Autodesk Inventor part; units mm, degrees
ref_plane "YZ Plane" through (0, 0, 0) normal (1, 0, 0) x (0, 1, 0)
ref_plane "XZ Plane" through (0, 0, 0) normal (0, 1, 0) x (-1, 0, 0)
ref_plane "XY Plane" through (0, 0, 0) normal (0, 0, 1) x (1, 0, 0)
sketch "Sketch1" plane through (0, 0, 0) normal (0, 0, 1) x (1, 0, 0)
  arc A0 (62.3383, -89.7392) -> (-62.3386, -89.7387) centre (0.0001, -5.2464) ccw
  arc A1 (61.8662, -89.0928) -> (-61.866, -89.0928) centre (0.0001, -5.2464) ccw
  line L0 (-62.3386, -89.7387) -> (-61.866, -89.0928)
  line L1 (62.3383, -89.7392) -> (61.8662, -89.0928)
  point P0 (0, 0)
  dimension "d0" = 208.4
extrude "Extrusion1" add sketch "Sketch1" along normal blind 30
ref_plane "Work Plane1" through (61.0727, -89.6701, 0) normal (0.6382, -0.7699, 0) x (0.7699, 0.6382, 0)
sketch "Sketch2" plane through (61.0727, -89.6701, 0) normal (0.6382, -0.7699, 0) x (0.7699, 0.6382, 0)
  circle A0 centre (6.5, 25.5) radius 1.4
  circle A1 centre (6.5, 4.5) radius 1.4
  point P0 (10.2035, 0)
extrude "Extrusion2" cut sketch "Sketch2" along normal blind 30
mirror "Mirror1" about plane through (0, 0, 0) normal (1, 0, 0) of "Extrusion2"
properties part number "3rdShroud"
Model file for the job. Use its own axes, mm. Give positions to 0.01 mm unless a question says otherwise; leave off trailing zeros. Loops run counter-clockwise (first coordinate to the right, second up) from the corner with the lowest first, then second, coordinate; pieces in that order, holes last.
Item 1: Slice it at D-D (x = 42.5). Write the cut outline in (y, z).
Check values:
outline: (89.89, 0) - (90.77, 0) - (90.77, 30) - (89.89, 30) - close
Item 2: Drop flat-ended pins along their axis: P1, Ø1, axis at x = -81.5, z = 23.5, coming from the -Y side; P2, Ø3, axis at y = 5.5, z = 19.5, coming from the -X side; P3, Ø8, axis at y = 4.5, z = 5.5, coming from the -X side. Give the stop position or say it passes through.
Check values:
P1: stops at y = -72.06
P2: stops at x = -104.59
P3: stops at x = -104.84
Item 3: Slice it at B-B (y = 35.5). Write the cut outline in (x, z).
Check values:
outline: (-96.77, 0) - (-95.9, 0) - (-95.9, 30) - (-96.77, 30) - close; (95.9, 0) - (96.77, 0) - (96.77, 30) - (95.9, 30) - close
Item 4: Mould opens along X. For faces 1 (the face through (-3.65, 98.89, 14.79)), 2 (the face through (-3.68, 99.69, 14.79)) say: +X half, -X half, draft (parallel to the pull), parting line (faces both ways), or undercut.
Check values:
face 1: undercut
face 2: parting line
Item 5: Drill centre lines: line 1 along Y through (x, z) = (94.5, 21.5); line 2 along Y through (x, z) = (86.5, 5); line 3 along X through (y, z) = (59.5, 3). Where is each one in solid material? Low to high.
Check values:
line 1: y = -51.02 to -49.15, 38.66 to 40.52
line 2: y = -64.77 to -63.34, 52.85 to 54.28
line 3: x = -82.66 to -81.64, 81.64 to 82.66
Item 6: Slice it at A-A (y = 54.5). Write the cut outline in (x, z).
Check values:
outline: (-86.34, 0) - (-85.37, 0) - (-85.37, 30) - (-86.34, 30) - close; (85.37, 0) - (86.35, 0) - (86.35, 30) - (85.37, 30) - close
Item 7: Slice it at C-C (z = 15.5). Write the cut outline in (x, y), plus the area to 3 significant figures.
Check values:
outline: (-62.34, -89.74) - (-61.87, -89.09) arc R104.2 cw (long way) to (61.87, -89.09) - (62.34, -89.74) arc R105 ccw (long way) to start
area: 420 mm2
